The listing builds one solid part. Answer for the finished solid, in the listing's coordinates (mm). Give positions to 0.01 mm unless a question says otherwise; leave off trailing zeros. Write each loop counter-clockwise with the first axis right and the second up, starting at its lowest first coordinate (ties: lowest second). Pieces come first, ordered by that corner, then holes. Notation, with made-up numbers: M 32.5,-12 L 37.5,-12 A3 cw 37.5,-7 Z; hole C 14,-0.75 d8. An arc over 180 degrees is marked long. Return JSON: item names as keys, results as strings.
from build123d import *

# Parameters (mm, degrees)
F1_DEPTH = 300


with BuildPart() as f1:
    # F0 (on Front) → F1 (new body, symmetric)
    with BuildSketch(Plane.XZ):
        with BuildLine():
            Line((100, 0), (0, 0))
            Line((0, 0), (0, -200))
            Line((0, -200), (200, -200))
            Line((200, -200), (200, -100))
            ThreePointArc((200, -100), (170.710678, -29.289322), (100, 0))
        make_face()
    extrude(amount=F1_DEPTH, both=True)


solid = f1.part
Item 1: Given pin 1 Ø8 at (y, z) = (129, -177) entering from -X, flat-ended and moving along its own axis, determine where the tip first touches the part or whether it passes through.
Geometry results:
{"pin 1": "stops at x = 0"}
Item 2: Find the intervals of material crossed by line 1 (X direction, y = -123, z = -99.5); line 2 (X direction, y = 102, z = -49); line 3 (Z direction, x = 121.5, y = -61), in increasing order.
Geometry results:
{"line 1": "x = 0 to 200", "line 2": "x = 0 to 186.02", "line 3": "z = -200 to -2.34"}
Item 3: A cutting plane is placed at A-A, the plane y = 177. Write down the section's boundary in (x, z), plus the area to 3 significant figures.
Geometry results:
{"outline": "M 0,-200 L 200,-200 L 200,-100 A100 ccw 100,0 L 0,0 Z", "area": "37,900 mm2"}
Item 4: A cutting plane is placed at B-B, the plane x = 175.5. Write down the section's boundary in (y, z).
Geometry results:
{"outline": "M -300,-200 L 300,-200 L 300,-34.43 L -300,-34.43 Z"}
Item 5: A cutting plane is placed at C-C, the plane x = 146. Write down the section's boundary in (y, z), plus the area to 3 significant figures.
Geometry results:
{"outline": "M -300,-200 L 300,-200 L 300,-11.21 L -300,-11.21 Z", "area": "113,000 mm2"}
